Verification items for this drawing (mm, ordinates from the low corner). Coordinates: 2 decimals unless noted, no trailing zeros. Order: outer loops, then holes, each group sorted by start corner. A loop starts at its lowest first (then second) coordinate and runs counter-clockwise, first axis right, second up. Notation, with made-up numbers: M 40.5,-30.75 L 66.5,-30.75 A23 ccw 66.5,6.25 Z; hole C -17.5,21.5 d1. An arc over 180 degrees is marked long. Answer as a JSON object with one key per item and string values. Group by question number.
(1) Cross-section at D-D (z = 2). Enter the section's corners in (x, y), plus the area to 3 significant figures.
(2) Gauge pin test, flat end, axial feed: pin 1 Ø6.5 at (x, y) = (78, 23.5) entering from +Z. Record the tip position at first contact, or that the pin passes through.
(3) Cross-section at C-C (y = 23.5). Enter the section's corners in (x, z), plus the area to 3 significant figures.
(4) Cross-section at B-B (y = 41). Enter the section's corners in (x, z).
(5) Material ranges on line 1 (Y direction, x = 13, z = 5.65); line 2 (Y direction, x = 78, z = 4.55); line 3 (X direction, y = 43, z = 5.15), recorded low to high.
(6) Cross-section at A-A (x = 13). Enter the section's corners in (y, z).
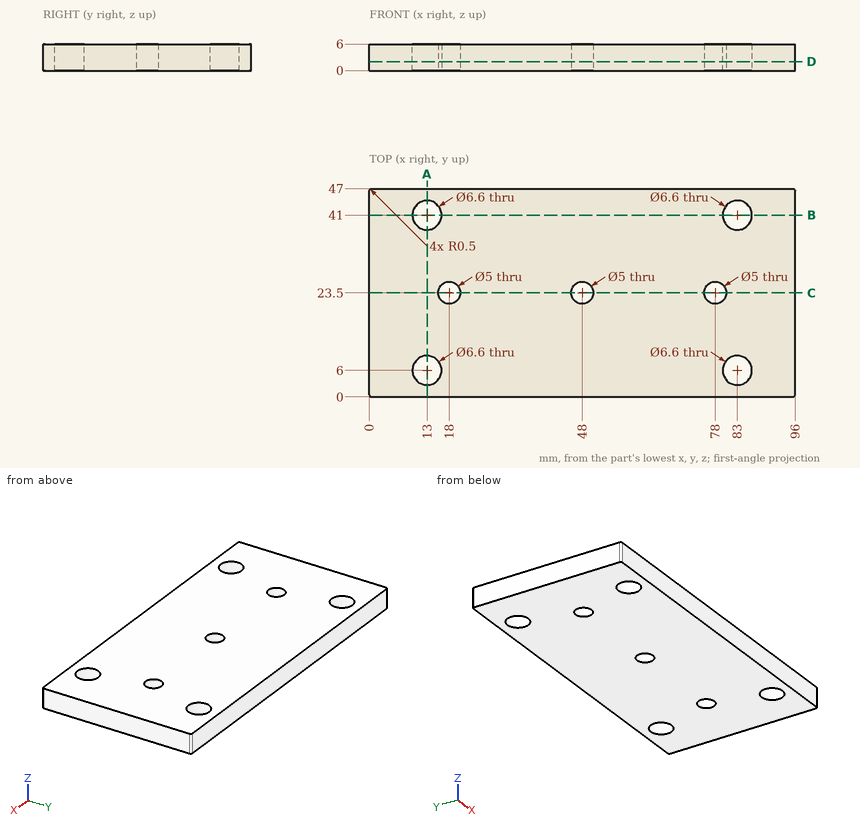
Taken from the geometry:
{
 "1": {"outline": "M 0,0.5 A0.5 ccw 0.5,0 L 95.5,0 A0.5 ccw 96,0.5 L 96,46.5 A0.5 ccw 95.5,47 L 0.5,47 A0.5 ccw 0,46.5 Z; hole C 13,6 d6.6; hole C 13,41 d6.6; hole C 18,23.5 d5; hole C 48,23.5 d5; hole C 78,23.5 d5; hole C 83,6 d6.6; hole C 83,41 d6.6", "area": "4,320 mm²"},
 "2": {"pin 1": "stops at z = 6"},
 "3": {"outline": "M 0,0 L 15.5,0 L 15.5,6 L 0,6 Z; M 20.5,0 L 45.5,0 L 45.5,6 L 20.5,6 Z; M 50.5,0 L 75.5,0 L 75.5,6 L 50.5,6 Z; M 80.5,0 L 96,0 L 96,6 L 80.5,6 Z", "area": "486 mm²"},
 "4": {"outline": "M 0,0 L 9.7,0 L 9.7,6 L 0,6 Z; M 16.3,0 L 79.7,0 L 79.7,6 L 16.3,6 Z; M 86.3,0 L 96,0 L 96,6 L 86.3,6 Z"},
 "5": {"line 1": "y = 0 to 2.7, 9.3 to 37.7, 44.3 to 47", "line 2": "y = 0 to 21, 26 to 47", "line 3": "x = 0 to 10.38, 15.62 to 80.38, 85.62 to 96"},
 "6": {"outline": "M 0,0 L 2.7,0 L 2.7,6 L 0,6 Z; M 9.3,0 L 37.7,0 L 37.7,6 L 9.3,6 Z; M 44.3,0 L 47,0 L 47,6 L 44.3,6 Z"}
}
